Could you check a few things on this drawing? It's one solid part, dimensions in mm from its lowest x, y, z. Give positions to 0.01 mm unless a question says otherwise; leave off trailing zeros. Write each loop counter-clockwise with the first axis right and the second up, starting at its lowest first coordinate (ties: lowest second). Pieces come first, ordered by that corner, then holes. Notation, with made-up numbers: M 15.25,13 L 44.25,13 A5 cw 44.25,20 Z; hole C 34,-30 d10. An arc over 180 degrees is marked long. Answer as CSV lines item,"result". Start each with the question number.
Q1. Thinking about a two-plate mould opening in Y: for the marked faces 1, 2 and 3, which applies, +Y half, -Y half, draft (parallel to the pull), parting line (faces both ways), or undercut?
Q2. Suppose I cut it at A-A (z = 2.4). Write out the boundary of the cut face in (x, y).
Q3. If I drill on line 1 along X through (y, z) = (14.25, 2.95); line 2 along X through (y, z) = (15, 2.45); line 3 along X through (y, z) = (8, 2.75), over which ranges is the centre line in solid material (lowest first)?
Q4. For pin 1 (1 mm diameter, centred on y = 20, z = 0.5, fed in from -X); pin 2 (1 mm diameter, centred on x = 21, z = 1, fed in from +Y); pin 3 (1.6 mm diameter, centred on x = 24.5, y = 14.5, fed in from +Z), each with a flat end and sliding along its axis, tell me the tip position at first contact or that it passes through.
Q5. Suppose I cut it at B-B (x = 14.5). Write out the boundary of the cut face in (y, z), then the cut area to 3 significant figures.
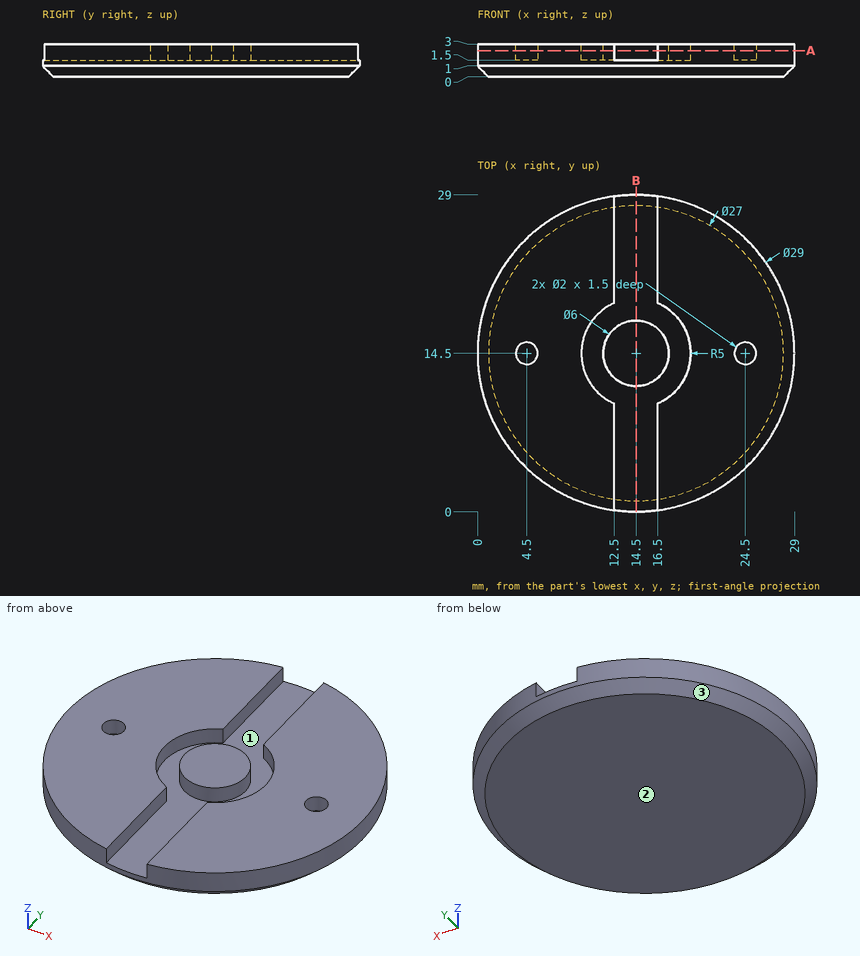
Resolved:
1,face 1,"undercut"
1,face 2,"draft"
1,face 3,"parting line"
2,outline,"C 14.5,14.5 d6; M 12.5,0.14 L 12.5,9.92 A5 cw 12.5,19.08 L 12.5,28.86 A14.5 ccw Z; M 16.5,0.14 A14.5 ccw 16.5,28.86 L 16.5,19.08 A5 cw 16.5,9.92 Z; hole C 4.5,14.5 d2; hole C 24.5,14.5 d2"
3,line 1,"0 to 3.53, 5.47 to 9.51, 11.51 to 17.49, 19.49 to 23.53, 25.47 to 29"
3,line 2,"0.01 to 3.63, 5.37 to 9.53, 11.54 to 17.46, 19.47 to 23.63, 25.37 to 28.99"
3,line 3,"1.54 to 12.5, 16.5 to 27.46"
4,pin 1,"x = 1.05"
4,pin 2,"y = 27.7"
4,pin 3,"z = 1.5"
5,outline,"M 0,1 L 1,0 L 28,0 L 29,1 L 29,1.5 L 17.5,1.5 L 17.5,3 L 11.5,3 L 11.5,1.5 L 0,1.5 Z"
5,area,"51.5 mm^2"
